Build history of the part. All positions in model axes, mm. A direction names the side the tool comes from. Round coordinates to 2 decimals unless told otherwise and drop trailing zeros. Write each loop counter-clockwise with the first axis right and the second up, starting at its lowest first coordinate (ties: lowest second). Pieces come first, ordered by that corner, then holes. Notation, with made-up numbers: (85, 39) - (121, 39) arc R17 cw to (121, 71) - close; hole circle Ø5 at (31, 75). An arc over 180 degrees is marked (long way). Write each question's results on one line, items separated by ' | '.
from build123d import *

# Parameters (mm, degrees)
VYSUNOUT_TENKOST_NN_1_DEPTH = 200
ODEBRAT_VYSUNUT_M1_REACH    = 241.596


with BuildPart() as part:
    # Skica1 → Vysunout tenkostěnný1 (new, symmetric)
    with BuildSketch(Plane(origin=(0, 0, 0), x_dir=(0, 0, -1), z_dir=(1, 0, 0))):
        with BuildLine():
            Line((-55, 22.5), (-62, 22.5))
            ThreePointArc((-62, 22.5), (-64.121320344, 21.621320344), (-65, 19.5))
            Line((-65, 19.5), (-65, -4.5))
            ThreePointArc((-65, -4.5), (-64.121320344, -6.621320344), (-62, -7.5))
            Line((-62, -7.5), (-31, -7.5))
            ThreePointArc((-31, -7.5), (-30.292893219, -7.792893219), (-30, -8.5))
            Line((-30, -8.5), (-30, -19.5))
            ThreePointArc((-30, -19.5), (-29.121320344, -21.621320344), (-27, -22.5))
            Line((-27, -22.5), (62, -22.5))
            ThreePointArc((62, -22.5), (64.121320344, -21.621320344), (65, -19.5))
            Line((65, -19.5), (65, 19.5))
            ThreePointArc((65, 19.5), (64.121320344, 21.621320344), (62, 22.5))
            Line((62, 22.5), (55, 22.5))
            Line((55, 22.5), (55, 20.5))
            Line((55, 20.5), (62, 20.5))
            ThreePointArc((62, 20.5), (62.707106781, 20.207106781), (63, 19.5))
            Line((63, 19.5), (63, -19.5))
            ThreePointArc((63, -19.5), (62.707106781, -20.207106781), (62, -20.5))
            Line((62, -20.5), (-27, -20.5))
            ThreePointArc((-27, -20.5), (-27.707106781, -20.207106781), (-28, -19.5))
            Line((-28, -19.5), (-28, -8.5))
            ThreePointArc((-28, -8.5), (-28.878679656, -6.378679656), (-31, -5.5))
            Line((-31, -5.5), (-62, -5.5))
            ThreePointArc((-62, -5.5), (-62.707106781, -5.207106781), (-63, -4.5))
            Line((-63, -4.5), (-63, 19.5))
            ThreePointArc((-63, 19.5), (-62.707106781, 20.207106781), (-62, 20.5))
            Line((-62, 20.5), (-55, 20.5))
            Line((-55, 20.5), (-55, 22.5))
        make_face()
    extrude(amount=VYSUNOUT_TENKOST_NN_1_DEPTH, both=True)

    # Odebrat vysunutím1: up to this face of the body (flat: up to its plane)
    odebrat_vysunut_m1_end = Plane(part.part.faces().sort_by_distance((0, 0, -65))[0])
    # Skica2 → Odebrat vysunutím1 (cut, up to the picked face)
    with BuildSketch(Plane.XY.offset(65), mode=Mode.PRIVATE) as odebrat_vysunut_m1_sk1:
        Polygon((-155, -22.5), (-200, 22.5), (-200, -22.5), align=None)
    odebrat_vysunut_m1_tool1 = split(extrude(odebrat_vysunut_m1_sk1.sketch, amount=-ODEBRAT_VYSUNUT_M1_REACH, mode=Mode.PRIVATE), bisect_by=odebrat_vysunut_m1_end, keep=Keep.BOTH, mode=Mode.PRIVATE)
    # Skica2 → Odebrat vysunutím1 (cut, up to the picked face)
    with BuildSketch(Plane.XY.offset(65), mode=Mode.PRIVATE) as odebrat_vysunut_m1_sk2:
        Polygon((200, 22.5), (200, -22.5), (155, -22.5), align=None)
    odebrat_vysunut_m1_tool2 = split(extrude(odebrat_vysunut_m1_sk2.sketch, amount=-ODEBRAT_VYSUNUT_M1_REACH, mode=Mode.PRIVATE), bisect_by=odebrat_vysunut_m1_end, keep=Keep.BOTH, mode=Mode.PRIVATE)
    add(odebrat_vysunut_m1_tool1.solids().sort_by(Axis((-185, -7.5, 65), (0, 0, -1)))[0], mode=Mode.SUBTRACT)
    add(odebrat_vysunut_m1_tool2.solids().sort_by(Axis((185, -7.5, 65), (0, 0, -1)))[0], mode=Mode.SUBTRACT)


solid = part.part
(1) Slice it at D-D, the plane z = 51.5. Write the cut outline in (x, y).
Worked answers:
outline: (-172, -5.5) - (-170, -7.5) - (170, -7.5) - (172, -5.5) - close
(2) Tool access for faces 5 (the flat face through (2, -22.5, -17)), 6 (the flat face through (3, 7, 63)), 7 (the flat face through (2, -14, 28)), 8 (the flat face through (2, -14, 30)), 9 (the flat face through (3, 0, -65)): list every direction of +Z, -Z, +X, -X, +Y, -Y with a clear straight run to the whole face (end or side of a thin tool).
Worked answers:
face 5: +Z, -Z, +X, -X, -Y | face 6: +X, -X | face 7: +X, -X, +Y | face 8: +Z, +X, -X, -Y | face 9: -Z, +X, -X, +Y, -Y
(3) Two-plate mould, pull along Y, no slides. Class faces 1 (the flat face through (3, 8, 65)), 2 (the flat face through (155.7, -21.8, 9.9)), 3 (the flat face through (3, 20.5, 59)), 4 (the flat face through (2, -5.5, 46)): released by +Y, released by -Y, zero draft, split by the parting line, or undercut.
Worked answers:
face 1: zero draft | face 2: released by -Y | face 3: undercut | face 4: undercut
(4) Slice it at C-C, the plane y = 15. Write the cut outline in (x, z), and give its area (3 significant figures).
Worked answers:
outline: (-192.5, -65) - (192.5, -65) - (192.5, -63) - (-192.5, -63) - close; (-192.5, 63) - (192.5, 63) - (192.5, 65) - (-192.5, 65) - close | area: 1,540 mm2
(5) Drill centre lines: probe 1 along Y at (x, z) = (26.5, -56.5); probe 2 along Z at (x, y) = (-74, 17); probe 3 along Z at (x, y) = (117, -13.5). Where is each one in solid material? Low to high. Write a range as [from, to].
Worked answers:
probe 1: y = [-22.5, -20.5], [20.5, 22.5] | probe 2: z = [-65, -63], [63, 65] | probe 3: z = [-65, -63], [28, 30]
(6) Slice it at B-B, the plane x = 118.5. Write the cut outline in (y, z), and give its area (3 significant figures).
Worked answers:
outline: (-22.5, -62) arc R3 ccw to (-19.5, -65) - (19.5, -65) arc R3 ccw to (22.5, -62) - (22.5, -55) - (20.5, -55) - (20.5, -62) arc R1 cw to (19.5, -63) - (-19.5, -63) arc R1 cw to (-20.5, -62) - (-20.5, 27) arc R1 cw to (-19.5, 28) - (-8.5, 28) arc R3 ccw to (-5.5, 31) - (-5.5, 62) arc R1 cw to (-4.5, 63) - (19.5, 63) arc R1 cw to (20.5, 62) - (20.5, 55) - (22.5, 55) - (22.5, 62) arc R3 ccw to (19.5, 65) - (-4.5, 65) arc R3 ccw to (-7.5, 62) - (-7.5, 31) arc R1 cw to (-8.5, 30) - (-19.5, 30) arc R3 ccw to (-22.5, 27) - close | area: 454 mm2
(7) Flat gauge pins, fed straight in: pin 1 Ø1.6 at (x, y) = (-99, 22) entering from +Z; pin 2 Ø1 at (x, y) = (-4, 21.5) entering from -Z; pin 3 Ø9 at (x, y) = (64, -16) entering from +Z. Where does each tip first touch, or does it go through?
Worked answers:
pin 1: stops at z = 64.47 | pin 2: stops at z = -64.6 | pin 3: stops at z = 30
(8) Slice it at A-A, the plane y = 0. Write the cut outline in (x, z), and give its area (3 significant figures).
Worked answers:
outline: (-177.5, -65) - (177.5, -65) - (177.5, -63) - (-177.5, -63) - close; (-177.5, 63) - (177.5, 63) - (177.5, 65) - (-177.5, 65) - close | area: 1,420 mm2
